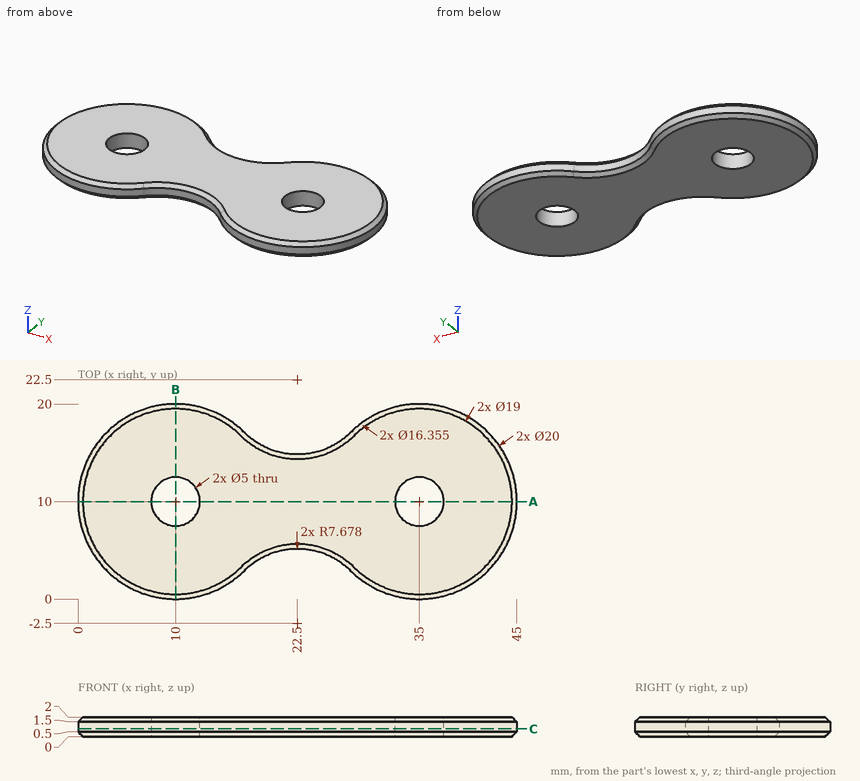
Here's the drawing with two shaded views (mm, measured from the low corner). I have some questions. Coordinates: 2 decimals unless noted, no trailing zeros. Loops run counter-clockwise (first coordinate to the right, second up) from the corner with the lowest first, then second, coordinate; pieces in that order, holes last. Notation, with made-up numbers: M 54,-19.5 L 61,-19.5 A21 ccw 61,8.5 Z; hole C 75,81 d9. An arc over 180 degrees is marked long. Put each result on its own line as item: value. Start each with the question number.
(1) Imagine slicing it at C-C on z = 0.8. List the corners of the cut face in (x, y) for me (1 decimal).
(2) I need wall thicknesses on probe 1 along X at (y, z) = (8.25, 0.7) (1 decimal); probe 2 along Y at (x, z) = (35, 0.95); probe 3 along X at (y, z) = (11.25, 1.4) (1 decimal). Which ranges of each line are inside material? Lowest first, please.
(3) Imagine slicing it at A-A on y = 10. List the corners of the cut face in (x, z) for me.
(4) Will this pin go through, and if not, where does the flat tip stop? pin 1 Ø1 at (x, z) = (24.5, 1) entering from +Y.
(5) Imagine slicing it at B-B on x = 10. List the corners of the cut face in (y, z) for me.
Worked answers:
1. outline: M 17.1,2.9 A7.7 cw 27.9,2.9 A10 ccw long 27.9,17.1 A7.7 cw 17.1,17.1 A10 ccw long Z; hole C 10,10 d5; hole C 35,10 d5
2. probe 1: x = 0.2 to 8.2, 11.8 to 33.2, 36.8 to 44.8
2. probe 2: y = 0 to 7.5, 12.5 to 20
2. probe 3: x = 0.1 to 7.8, 12.2 to 32.8, 37.2 to 44.9
3. outline: M 0,0.5 L 0.5,0 L 7.5,0 L 7.5,2 L 0.5,2 L 0,1.5 Z; M 12.5,0 L 32.5,0 L 32.5,2 L 12.5,2 Z; M 37.5,0 L 44.5,0 L 45,0.5 L 45,1.5 L 44.5,2 L 37.5,2 Z
4. pin 1: stops at y = 15.24
5. outline: M 0,0.5 L 0.5,0 L 7.5,0 L 7.5,2 L 0.5,2 L 0,1.5 Z; M 12.5,0 L 19.5,0 L 20,0.5 L 20,1.5 L 19.5,2 L 12.5,2 Z
